For this review, use the dimensioned drawing (mm, ordinates from the lowest corner) and the shaded views. A direction names the side the tool comes from. Coordinates: 2 decimals unless noted, no trailing zeros. Loops run counter-clockwise (first coordinate to the right, second up) from the corner with the lowest first, then second, coordinate; pieces in that order, holes last. Notation, with made-up numbers: (67, 77.5) - (107, 77.5) arc R14 ccw to (107, 91.5) - close; hole circle Ø3 at (56.25, -9.75). An arc over 180 degrees is marked (long way). Answer in a Markdown table with one row per item. Add a question column.
(1) To check wall thickness, follow L1, parallel to Z at x = 6.55, y = 2.75; L2, parallel to Z at x = 8.25, y = 7.5. State the ranges of each line that lie inside material, in increasing order. Write a range as [from, to].
(2) We need section B-B, the plane y = 2.75. Write out the cut boundary in (x, z), plus the area to 3 significant figures.
(3) We need section A-A, the plane z = 4.1. Write out the cut boundary in (x, y).
(4) We need section C-C, the plane x = 7.25. Write out the cut boundary in (y, z).
(5) We need section D-D, the plane z = 2.75. Write out the cut boundary in (x, y).
(6) Clearance check with flat-ended pins moving along their axes: pin 1 (1.6 mm diameter, centred on x = 9.5, y = 8, fed in from +Z); pin 2 (3 mm diameter, centred on y = 8.5, z = 3, fed in from -X); pin 3 (3 mm diameter, centred on x = 4.5, y = 8.5, fed in from -Z); pin 4 (1.6 mm diameter, centred on x = 8.5, y = 7.5, fed in from -Z). State where each tip first meets the part, or that it passes through.
(7) For the marked faces 1, 2 and 3, list the 3-axis set-ups (+Z, -Z, +X, -X, +Y, -Y) from which the entire face can be reached by the end or side of a thin tool; tool diameter is ignored.
(8) The part is to be moulded in two halves that separate along Z. For the marked faces 4, 5 and 6, say which applies: released by +Z, released by -Z, zero draft, split by the parting line, or undercut.
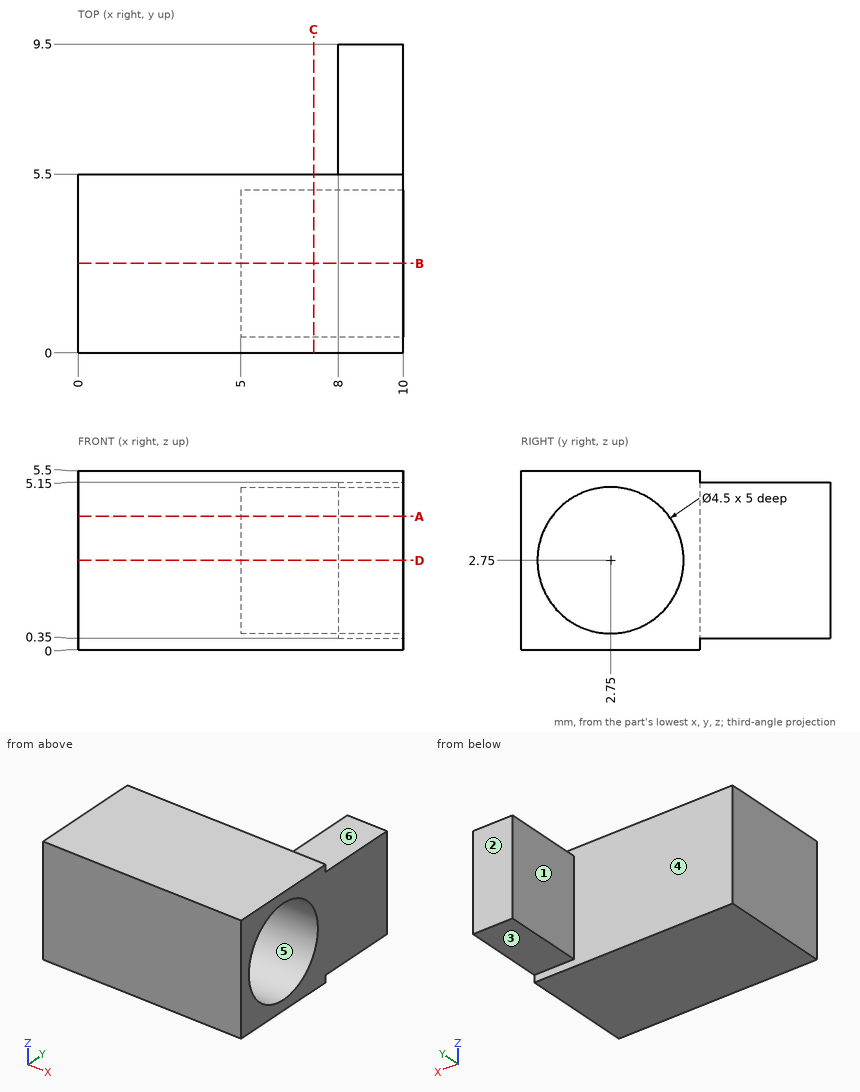
Responses:
| question | item | result |
|---|---|---|
| 1 | L1 | z = [0, 0.5], [5, 5.5] |
| 1 | L2 | z = [0.35, 5.15] |
| 2 | outline | (0, 0) - (10, 0) - (10, 0.5) - (5, 0.5) - (5, 5) - (10, 5) - (10, 5.5) - (0, 5.5) - close |
| 2 | area | 32.5 mm2 |
| 3 | outline | (0, 0) - (10, 0) - (10, 0.95) - (5, 0.95) - (5, 4.55) - (10, 4.55) - (10, 9.5) - (8, 9.5) - (8, 5.5) - (0, 5.5) - close |
| 4 | outline | (0, 0) - (5.5, 0) - (5.5, 5.5) - (0, 5.5) - close; hole circle Ø4.5 at (2.75, 2.75) |
| 5 | outline | (0, 0) - (10, 0) - (10, 0.5) - (5, 0.5) - (5, 5) - (10, 5) - (10, 9.5) - (8, 9.5) - (8, 5.5) - (0, 5.5) - close |
| 6 | pin 1 | stops at z = 5.15 |
| 6 | pin 2 | stops at x = 8 |
| 6 | pin 3 | passes through |
| 6 | pin 4 | stops at z = 0.35 |
| 7 | face 1 | +Z, -Z, -X, +Y |
| 7 | face 2 | +Z, -Z, +X, -X, +Y |
| 7 | face 3 | -Z, +X, -X, +Y |
| 8 | face 4 | zero draft |
| 8 | face 5 | undercut |
| 8 | face 6 | released by +Z |
